Work out the finished part from the listing and answer in its coordinate system (mm). A direction names the side the tool comes from. Give positions to 0.01 mm unless a question says otherwise; leave off trailing zeros. Loops run counter-clockwise (first coordinate to the right, second up) from the corner with the lowest first, then second, coordinate; pieces in that order, holes last.
from build123d import *

# Parameters (mm, degrees)
SKETCH1_W           = 19.05
SKETCH1_H           = 12.7
BOSS_EXTRUDE1_DEPTH = 3
SKETCH2_W           = 6
SKETCH2_H           = 12.7
BOSS_EXTRUDE2_DEPTH = 6
SKETCH3_W           = 12.319
SKETCH3_H           = 5.999999938
CUT_EXTRUDE1_DEPTH  = 17.710718865
FILLET1_R           = 1.5875


with BuildPart() as part:
    # Sketch1 → Boss-Extrude1 (new, symmetric)
    with BuildSketch(Plane(origin=(0, 0, 0), x_dir=(0, 0, -1), z_dir=(1, 0, 0))):
        Rectangle(SKETCH1_W, SKETCH1_H)
    extrude(amount=BOSS_EXTRUDE1_DEPTH, both=True)

    # Sketch2 → Boss-Extrude2 (add)
    with BuildSketch(Plane(origin=(0, 6.35, 0), x_dir=(1, 0, 0), z_dir=(0, 1, 0))):
        Rectangle(SKETCH2_W, SKETCH2_H)
    extrude(amount=BOSS_EXTRUDE2_DEPTH)

    # Sketch3 → Cut-Extrude1 (cut, through all)
    with BuildSketch(Plane(origin=(3, 0, 0), x_dir=(0, 0, -1), z_dir=(1, 0, 0))):
        Rectangle(SKETCH3_W, SKETCH3_H)
    extrude(amount=-CUT_EXTRUDE1_DEPTH, mode=Mode.SUBTRACT)

    # Fillet1
    fillet1_edges = [part.edges().sort_by_distance(p)[0] for p in [
        (0, 12.35, -6.35),
        (0, 12.35, 6.35),
    ]]
    fillet(fillet1_edges, radius=FILLET1_R)


solid = part.part
Item 1: For faces 1 (the face through (0, 6.35, 8)), 2 (the face through (0, -3, 0)), 3 (the face through (0, 9, -6.35)), 4 (the face through (0, 0, -9.525)), determine the directions among +Z, -Z, +X, -X, +Y, -Y from which every point of the face is accessible in a straight line to the end or side of a thin tool.
Item 2: Flat-ended cylindrical pins translate along their axes: pin 1 Ø3.5 at (x, y) = (-1.5, 8.5) entering from +Z; pin 2 Ø3.5 at (x, y) = (-0.5, 8) entering from -Z (3 decimals); pin 3 Ø1 at (x, z) = (-1, -8.5) entering from +Y. Find the tip coordinate at first contact, or state that the pin passes through.
Item 3: Determine the mould class of faces 5 (the face through (0, 0, -6.16)), 6 (the face through (3, 5, 0)), 7 (the face through (0, -6.35, 0)), 8 (the face through (0, 12.35, 0)) for opening direction Y: released by +Y, released by -Y, zero draft, split by the parting line, or undercut.
Item 4: Consider line 1 (Y direction, x = 2.15, z = 0.5); line 2 (Z direction, x = -1.7, y = 0.75) (1 decimal); line 3 (Z direction, x = 2.5, y = 9.25). Determine where each line is inside the solid, lowest interval first.
Item 5: Find section B-B, the plane y = -0.5. Write down the section's boundary in (x, z) (1 decimal).
Item 6: Find section A-A, the plane z = -0.5. Write down the section's boundary in (x, y).
Item 7: Find section D-D, the plane y = 8.5. Write down the section's boundary in (x, z), plus the area to 3 significant figures.
Ans:
1. face 1: +Z, +X, -X, +Y
1. face 2: +X, -X
1. face 3: -Z, +X, -X, +Y
1. face 4: -Z, +X, -X, +Y, -Y
2. pin 1: stops at z = 6.35
2. pin 2: stops at z = -9.525
2. pin 3: stops at y = 6.35
3. face 5: undercut
3. face 6: zero draft
3. face 7: released by -Y
3. face 8: released by +Y
4. line 1: y = -6.35 to -3, 3 to 12.35
4. line 2: z = -9.5 to -6.2, 6.2 to 9.5
4. line 3: z = -6.35 to 6.35
5. outline: (-3, -9.5) - (3, -9.5) - (3, -6.2) - (-3, -6.2) - close; (-3, 6.2) - (3, 6.2) - (3, 9.5) - (-3, 9.5) - close
6. outline: (-3, -6.35) - (3, -6.35) - (3, -3) - (-3, -3) - close; (-3, 3) - (3, 3) - (3, 12.35) - (-3, 12.35) - close
7. outline: (-3, -6.35) - (3, -6.35) - (3, 6.35) - (-3, 6.35) - close
7. area: 76.2 mm2
